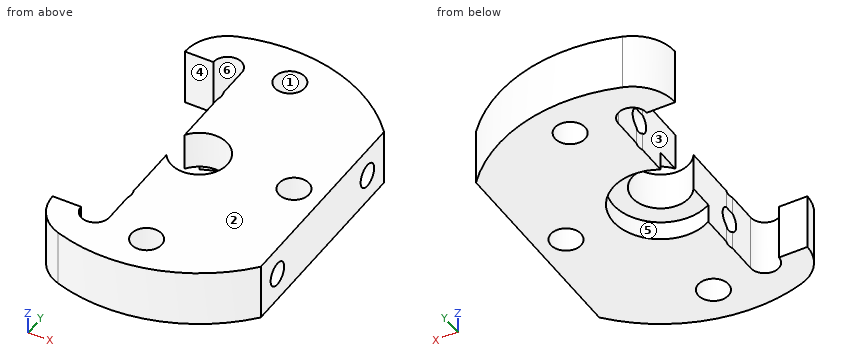
Autodesk Inventor part; units mm, degrees
ref_plane "YZ Plane" through (0, 0, 0) normal (1, 0, 0) x (0, 1, 0)
ref_plane "XZ Plane" through (0, 0, 0) normal (0, 1, 0) x (-1, 0, 0)
ref_plane "XY Plane" through (0, 0, 0) normal (0, 0, 1) x (1, 0, 0)
sketch "スケッチ1" plane through (0, 0, 0) normal (0, 0, 1) x (1, 0, 0)
  arc A0 (-2.5, -4.3301) -> (-2.5, 4.3301) centre (0, 0) ccw construction
  arc A1 (-5.423, -16.2691) -> (-5.423, 16.2691) centre (0, 0) ccw
  arc A2 (-2.5, -1.6583) -> (-2.5, 1.6583) centre (0, 0) ccw
  line L0 (-2.5, -12) -> (-2.5, -1.6583)
  line L1 (-2.5, 1.6583) -> (-2.5, 12)
  line L2 (-8.5, -12) -> (-2.5, -12)
  line L3 (-2.5, -12) -> (-2.5, 12)
  line L4 (-2.5, 12) -> (-8.5, 12)
  line L5 (-8.5, 12) -> (-8.5, -12)
  line L6 (-8.5, -12) -> (-2.5, 12) construction
  line L7 (-2.5, -12) -> (-8.5, 12) construction
  line L8 (6.2704, -6.6573) -> (-2.5, -6.6573) construction
  line L9 (-2.5, -6.6573) -> (-2.5, -9.6573) construction
  line L10 (-2.5, -9.6573) -> (6.2704, -9.6573) construction
  line L11 (6.2704, -9.6573) -> (6.2704, -6.6573) construction
  arc A3 (-5.5, -12) -> (-2.5, -12) centre (-4, -12) ccw
  arc A4 (-2.5, 12) -> (-5.5, 12) centre (-4, 12) ccw
  arc A5 (-8.5, -12) -> (-5.423, -16.2691) centre (-4, -12) ccw
  arc A6 (-5.423, 16.2691) -> (-8.5, 12) centre (-4, 12) ccw
  point P0 (-5.5, 0)
  point P1 (-5.5, 0)
  point P2 (-2.5, 13.775)
  point P3 (-2.5, -13.775)
  dimension "d0" = 10
  dimension "d2" = 6
  dimension "d9" = 2.5
  dimension "d10" = 6
  dimension "d11" = 24
  dimension "d12" = 3
  dimension "d14" = 1.5
  dimension "d15" = 3
  dimension "d16" = 3
extrude "押し出し1" add sketch "スケッチ1" along normal blind 6 contours A5 L2 A3 L0 A2 L1 A4 L4 A6 A1
sketch "スケッチ2" plane through (0, 0, 0) normal (0, 0, -1) x (-1, 0, 0)
  circle A0 centre (0, 0) radius 5
  dimension "d6" = 10
extrude "押し出し2" cut sketch "スケッチ2" against normal blind 2
sketch "スケッチ4" plane through (0, 0, 0) normal (0, 0, -1) x (-1, 0, 0)
  arc A0 (2.5, 4.3301) -> (2.5, -4.3301) centre (0, 0) ccw
  line L0 (2.5, 4.3301) -> (2.5, 12)
  arc A1 (5.5, 12) -> (2.5, 12) centre (4, 12) ccw
  line L1 (5.5, 12) -> (8.5, 12)
  arc A2 (8.5, 12) -> (5.423, 16.2691) centre (4, 12) ccw
  arc A3 (5.423, 16.2691) -> (5.423, -16.2691) centre (0, 0) ccw
  arc A4 (5.423, -16.2691) -> (8.5, -12) centre (4, -12) ccw
  line L2 (8.5, -12) -> (5.5, -12)
  arc A5 (2.5, -12) -> (5.5, -12) centre (4, -12) ccw
  line L3 (2.5, -12) -> (2.5, -4.3301)
  arc A6 (2.5, -7.6265) -> (2.5, -8.7036) centre (3.9, -8.1651) ccw
  arc A7 (2.5, 8.7036) -> (2.5, 7.6265) centre (3.9, 8.1651) ccw
  point P0 (2.4, 8.1651)
  point P1 (2.5, 8.1651)
  point P2 (2.4, -8.1651)
  point P3 (2.5, -8.1651)
  dimension "d17" = 1.5
  dimension "d18" = 0.1
extrude "押し出し3" cut sketch "スケッチ4" against normal through all contours A7 L0 | L3 A6
sketch "スケッチ5" plane through (0, 0, 0) normal (0, 0, -1) x (-1, 0, 0)
  arc A0 (2.5, -7.6265) -> (2.5, -8.7036) centre (3.9, -8.1651) ccw
  line L0 (2.5, -7.6265) -> (2.5, -4.3301)
  arc A1 (2.5, 4.3301) -> (2.5, -4.3301) centre (0, 0) ccw
  line L1 (2.5, 4.3301) -> (2.5, 7.6265)
  arc A2 (2.5, 8.7036) -> (2.5, 7.6265) centre (3.9, 8.1651) ccw
  line L2 (2.5, 8.7036) -> (2.5, 12)
  arc A3 (5.5, 12) -> (2.5, 12) centre (4, 12) ccw
  line L3 (5.5, 12) -> (8.5, 12)
  arc A4 (8.5, 12) -> (5.423, 16.2691) centre (4, 12) ccw
  arc A5 (5.423, 16.2691) -> (5.423, -16.2691) centre (0, 0) ccw
  arc A6 (5.423, -16.2691) -> (8.5, -12) centre (4, -12) ccw
  line L4 (8.5, -12) -> (5.5, -12)
  arc A7 (2.5, -12) -> (5.5, -12) centre (4, -12) ccw
  line L5 (2.5, -12) -> (2.5, -8.7036)
  line L6 (3.9, -8.1651) -> (-13, -8.1651) construction
  line L7 (3.9, 8.1651) -> (-13, 8.1651) construction
  line L8 (-13, -11.1845) -> (-13, 11.1845)
  circle A8 centre (-10, 0) radius 1.6
  circle A9 centre (-2, -13) radius 1.6
  circle A10 centre (-2, 13) radius 1.6
  line L9 (-2, -13) -> (-2, 13)
  point P0 (-2, 0)
  dimension "d21" = 13
  dimension "d22" = 3.2
  dimension "d23" = 10
  dimension "d24" = 3.2
  dimension "d25" = 3.2
  dimension "d26" = 26
  dimension "d27" = 2
extrude "押し出し4" cut sketch "スケッチ5" against normal through all contours A9 | A10 | A5 L8 | A8
sketch "スケッチ6" plane through (13, -11.1845, 0) normal (1, 0, 0) x (0, 0, -1)
  line L0 (0, 3.5579) -> (0, 2.4809)
  line L1 (0, 19.888) -> (0, 18.811)
  line L2 (0, 19.3495) -> (-3, 19.3495)
  line L3 (0, 3.0194) -> (-3, 3.0194)
  point P0 (0, 11.1845)
  dimension "d30" = 3
hole "穴1" at (13, 8.1651, 3) at (13, -8.1651, 3) direction (-1, 0, 0) diameter 2.459 end through all
equation "\"d16\" = d15"
properties part number "D留め板"
Read the model definition and answer for the solid it produces. Units are mm, in the model's axes. Face numbers are marked on the shaded views. A direction names the side the tool comes from. Coordinates: 2 decimals unless noted, no trailing zeros. Write each loop counter-clockwise with the first axis right and the second up, starting at its lowest first coordinate (ties: lowest second). Pieces come first, ordered by that corner, then holes. Notation, with made-up numbers: (83, -40) -> (126, -40) arc R31 ccw to (126, -15) -> close; hole circle Ø2 at (16.25, 29). An arc over 180 degrees is marked (long way). Write item = value, one per line.
(1) Given pin 1 Ø3.5 at (y, z) = (-11, 3.5) entering from -X; pin 2 Ø1.8 at (y, z) = (-5.5, 1.5) entering from -X; pin 3 Ø5.5 at (x, y) = (0, 0) entering from +Z; pin 4 Ø0.9 at (x, z) = (-7, 2.5) entering from -Y, each flat-ended and moving along its own axis, determine where each tip first touches the part or whether it passes through.
From the geometry:
pin_1 = -8.5
pin_2 = -2.5
pin_3 = through
pin_4 = -15.71
(2) Section B-B on x = 2 is taken. Write down the section's boundary in (y, z), plus the area to 3 significant figures.
From the geometry:
outline = (-17.03, 0) -> (-14.6, 0) -> (-14.6, 6) -> (-17.03, 6) -> close; (-11.4, 0) -> (-4.58, 0) -> (-4.58, 2) -> (-2.24, 2) -> (-2.24, 6) -> (-11.4, 6) -> close; (2.24, 2) -> (4.58, 2) -> (4.58, 0) -> (11.4, 0) -> (11.4, 6) -> (2.24, 6) -> close; (14.6, 0) -> (17.03, 0) -> (17.03, 6) -> (14.6, 6) -> close; hole circle Ø2.46 at (-8.17, 3); hole circle Ø2.46 at (8.17, 3)
area = 120 mm2
(3) Straight lines are drawn through the part: L1, parallel to Y at x = 2, z = 3; L2, parallel to Y at x = 2.25, z = 4; L3, parallel to Y at x = 2, z = 4.45. For each, find the intervals that lie inside material, in ascending order. Write a range as from..to.
From the geometry:
L1 = -17.03..-14.6, -11.4..-9.39, -6.94..-2.24, 2.24..6.94, 9.39..11.4, 14.6..17.03
L2 = -17..-14.58, -11.42..-8.88, -7.45..-1.98, 1.98..7.45, 8.88..11.42, 14.58..17
L3 = -17.03..-14.6, -11.4..-2.24, 2.24..11.4, 14.6..17.03
(4) Section C-C on x = 11 is taken. Write down the section's boundary in (y, z), plus the area to 3 significant figures.
From the geometry:
outline = (-13.16, 0) -> (-1.25, 0) -> (-1.25, 6) -> (-13.16, 6) -> close; (1.25, 0) -> (13.16, 0) -> (13.16, 6) -> (1.25, 6) -> close; hole circle Ø2.46 at (-8.17, 3); hole circle Ø2.46 at (8.17, 3)
area = 133 mm2
(5) Which of the six approach directions +Z, -Z, +X, -X, +Y, -Y give full straight-line access (tool end or side, diameter ignored) to the marked faces 4, 5 and 6?
From the geometry:
face_4 = +Z, -Z, -X
face_5 = -Z
face_6 = +Z, -Z
(6) For a pull along X with two mould halves and no side action, classify the marked faces 1, 2 and 3 as +X half, -X half, draft (parallel to the pull), parting line (faces both ways), or undercut.
From the geometry:
face_1 = undercut
face_2 = draft
face_3 = -X half
(7) Section A-A on y = 0 is taken. Write down the section's boundary in (x, z).
From the geometry:
outline = (3, 2) -> (5, 2) -> (5, 0) -> (8.4, 0) -> (8.4, 6) -> (3, 6) -> close; (11.6, 0) -> (13, 0) -> (13, 6) -> (11.6, 6) -> close
(8) Section D-D on z = 3 is taken. Write down the section's boundary in (x, y), plus the area to 3 significant figures.
From the geometry:
outline = (-8.5, -12) arc R4.5 ccw to (-5.42, -16.27) arc R17.15 ccw to (13, -11.18) -> (13, -9.39) -> (-2.5, -9.39) -> (-2.5, -12) arc R1.5 cw to (-5.5, -12) -> close; (-8.5, 12) -> (-5.5, 12) arc R1.5 cw to (-2.5, 12) -> (-2.5, 9.39) -> (13, 9.39) -> (13, 11.18) arc R17.15 ccw to (-5.42, 16.27) arc R4.5 ccw to start; (-2.5, -6.94) -> (13, -6.94) -> (13, 6.94) -> (-2.5, 6.94) -> (-2.5, 1.66) arc R3 cw (long way) to (-2.5, -1.66) -> close; hole circle Ø3.2 at (2, -13); hole circle Ø3.2 at (2, 13); hole circle Ø3.2 at (10, 0)
area = 396 mm2
